The listing builds one solid part. Answer for the finished solid, in the listing's coordinates (mm). Coordinates: 2 decimals unless noted, no trailing zeros. Loops run counter-clockwise (first coordinate to the right, second up) from the corner with the lowest first, then second, coordinate; pieces in that order, holes last. Notation, with made-up numbers: (51.25, 25) -> (68.25, 25) arc R23 cw to (68.25, 56) -> close; hole circle Ø11 at (-21.75, 54.25). An arc over 180 degrees is marked (long way). Answer in a Markdown table with one row per item.
```python
from build123d import *

# Parameters (mm, degrees)
F0_W     = 9.525
F0_H     = 3.175
F1_DEPTH = 12.7
F2_R     = 1.4605
F4_DEPTH = 25.4
F3_R     = 1.4605
F5_DEPTH = 25.4


with BuildPart() as f1:
    # F0 (on Top) → F1 (new body)
    with BuildSketch(Plane.XY):
        Polygon((-46.713472, 32.047768), (-46.713472, 19.347768), (-43.538472, 19.347768), (-43.538472, 28.872768), (-43.538472, 32.047768), align=None)
        with Locations((-38.775972, 30.460268)):
            Rectangle(F0_W, F0_H)
    extrude(amount=F1_DEPTH)

    # F2 (on face) → F4 (cut)
    with BuildSketch(Plane.XZ.offset(-28.872768)):
        with Locations((-38.775972, 6.35)):
            Circle(F2_R)
    extrude(amount=-F4_DEPTH, mode=Mode.SUBTRACT)

    # F3 (on face) → F5 (cut)
    with BuildSketch(Plane.YZ.offset(-43.538472)):
        with Locations((24.110268, 6.35)):
            Circle(F3_R)
    extrude(amount=-F5_DEPTH, mode=Mode.SUBTRACT)


solid = f1.part
```
Item 1: Find the intervals of material crossed by probe 1 along Y at (x, z) = (-42.75, 9); probe 2 along X at (y, z) = (24.25, 2.25); probe 3 along X at (y, z) = (29.5, 5.75), in increasing order.
Findings below:
| item | result |
|---|---|
| probe 1 | y = 28.87 to 32.05 |
| probe 2 | x = -46.71 to -43.54 |
| probe 3 | x = -46.71 to -40.11, -37.44 to -34.01 |
Item 2: A cutting plane is placed at A-A, the plane z = 6.35. Determine the outline of the cut face in (x, y).
Findings below:
| item | result |
|---|---|
| outline | (-46.71, 19.35) -> (-43.54, 19.35) -> (-43.54, 22.65) -> (-46.71, 22.65) -> close; (-46.71, 25.57) -> (-43.54, 25.57) -> (-43.54, 28.87) -> (-40.24, 28.87) -> (-40.24, 32.05) -> (-46.71, 32.05) -> close; (-37.32, 28.87) -> (-34.01, 28.87) -> (-34.01, 32.05) -> (-37.32, 32.05) -> close |
Item 3: A cutting plane is placed at B-B, the plane x = -44.25. Determine the outline of the cut face in (y, z).
Findings below:
| item | result |
|---|---|
| outline | (19.35, 0) -> (32.05, 0) -> (32.05, 12.7) -> (19.35, 12.7) -> close; hole circle Ø2.92 at (24.11, 6.35) |
Item 4: Flat-ended cylindrical pins translate along their axes: pin 1 Ø2 at (y, z) = (21.5, 7) entering from +X; pin 2 Ø1.8 at (x, z) = (-38.78, 6.35) entering from +Y; pin 3 Ø1 at (x, z) = (-41, 2.5) entering from -Y. Find the tip coordinate at first contact, or state that the pin passes through.
Findings below:
| item | result |
|---|---|
| pin 1 | stops at x = -43.54 |
| pin 2 | passes through |
| pin 3 | stops at y = 28.87 |
Item 5: A cutting plane is placed at D-D, the plane x = -38.25. Determine the outline of the cut face in (y, z), plus the area to 3 significant figures.
Findings below:
| item | result |
|---|---|
| outline | (28.87, 0) -> (32.05, 0) -> (32.05, 4.99) -> (28.87, 4.99) -> close; (28.87, 7.71) -> (32.05, 7.71) -> (32.05, 12.7) -> (28.87, 12.7) -> close |
| area | 31.7 mm2 |
Item 6: A cutting plane is placed at C-C, the plane y = 25. Determine the outline of the cut face in (x, z), plus the area to 3 significant figures.
Findings below:
| item | result |
|---|---|
| outline | (-46.71, 0) -> (-43.54, 0) -> (-43.54, 5.19) -> (-46.71, 5.19) -> close; (-46.71, 7.51) -> (-43.54, 7.51) -> (-43.54, 12.7) -> (-46.71, 12.7) -> close |
| area | 33.0 mm2 |
Item 7: Determine the mould class of faces 1 (the face through (-45.1, 25.46, 5.79)), 2 (the face through (-40, 28.873, 5)), 3 (the face through (-43.538, 25, 5)) for opening direction Y: +Y half, -Y half, draft (parallel to the pull), parting line (faces both ways), or undercut.
Findings below:
| item | result |
|---|---|
| face 1 | undercut |
| face 2 | -Y half |
| face 3 | draft |
